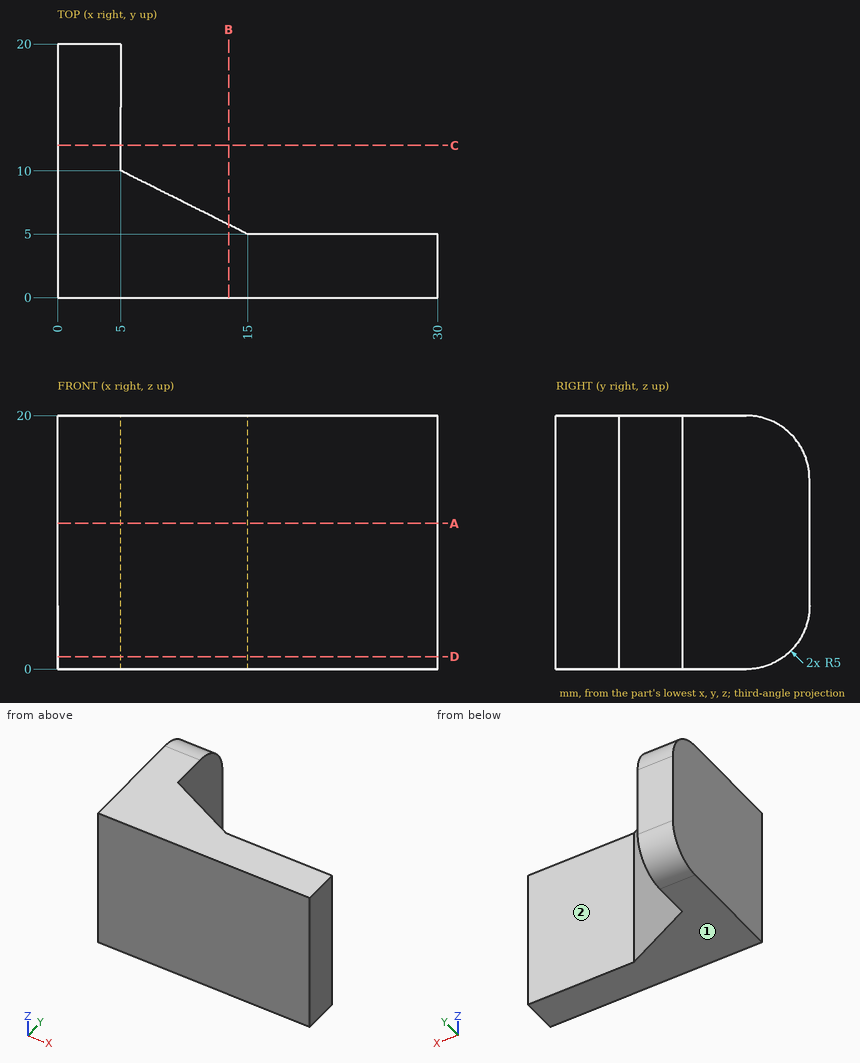
Geometry check sheet. Reference: drawing and pictorial views, mm from the part's lowest x, y, z. A direction names the side the tool comes from. Round coordinates to 2 decimals unless told otherwise and drop trailing zeros. Loops run counter-clockwise (first coordinate to the right, second up) from the corner with the lowest first, then second, coordinate; pieces in that order, holes last. Notation, with made-up numbers: (65, -12.5) - (124, -12.5) arc R21 ccw to (124, 23.5) - close; hole circle Ø7 at (-7, 75.25). An arc over 180 degrees is marked (long way). One line per question, with ' | ' between items. Start each with the question number.
1. Depth check by flat-ended pin: pin 1 (2 mm diameter, centred on x = 26, z = 3, fed in from +Y); pin 2 (11 mm diameter, centred on y = 16.5, z = 11.5, fed in from +X); pin 3 (10 mm diameter, centred on y = 11, z = 17.5, fed in from +X). Enter the tip coordinate at first touch or a pass-through.
2. Scan lines: line 1 (Y direction, x = 18, z = 18.5); line 2 (Y direction, x = 4.25, z = 15.5). Record each from-to range of solid material in increasing order. Write a range as [from, to].
3. Cross-section at A-A on z = 11.5. Record the cut outline in (x, y), then the cut area to 3 significant figures.
4. Tool access check on the marked faces 1 and 2. Record the directions out of +Z, -Z, +X, -X, +Y, -Y that give a thin tool (end or side, any length) a straight path to the whole face; none if there is none.
5. Cross-section at C-C on y = 12. Record the cut outline in (x, z).
6. Cross-section at D-D on z = 1. Record the cut outline in (x, y), then the cut area to 3 significant figures.
7. Cross-section at B-B on x = 13.5. Record the cut outline in (y, z).
Taken from the geometry:
1) pin 1: y = 5 | pin 2: x = 5 | pin 3: x = 13
2) line 1: [0, 5] | line 2: [0, 19.97]
3) outline: (0, 0) - (30, 0) - (30, 5) - (15, 5) - (5, 10) - (5, 20) - (0, 20) - close | area: 250 mm²
4) face 1: -Z, +X, -X, +Y, -Y | face 2: +Z, -Z, +X, +Y
5) outline: (0, 0) - (5, 0) - (5, 20) - (0, 20) - close
6) outline: (0, 0) - (30, 0) - (30, 5) - (15, 5) - (5, 10) - (5, 18) - (0, 18) - close | area: 240 mm²
7) outline: (0, 0) - (5.75, 0) - (5.75, 20) - (0, 20) - close
